```python
from build123d import *

# Parameters (mm, degrees)
SKETCH066_R     = 2.7
PAD030_DEPTH    = 10
SKETCH063_R     = 2.6
POCKET025_DEPTH = 8
SKETCH064_R     = 3
POCKET026_DEPTH = 1
SKETCH067_R     = 2
POCKET027_DEPTH = 8


with BuildPart() as loft003:
    # Sketch066 → Loft003 section 0
    with BuildSketch(Plane.XY.offset(18)):
        with Locations((-5, 0)):
            Circle(SKETCH066_R)
    # Sketch065 → Loft003 section 1
    with BuildSketch(Plane.XY.offset(38)):
        with BuildLine():
            ThreePointArc((-6, 1.5), (-7.5, 0), (-6, -1.5))
            Line((-6, -1.5), (-2, -1.5))
            ThreePointArc((-2, -1.5), (-0.5, 0), (-2, 1.5))
            Line((-2, 1.5), (-6, 1.5))
        make_face()
    loft()


with BuildPart() as part_mirroring003:
    # Part__Mirroring003: instance of Loft003
    add(loft003.part.mirror(Plane(origin=(0, 0, 0), x_dir=(0, -1, 0), z_dir=(1, 0, 0))))


with BuildPart() as fusion003:
    # Fusion003 base: copy of Loft003
    add(loft003.part)

    # Fusion003: union Part__Mirroring003
    add(part_mirroring003.part)


with BuildPart() as cut002:
    # Sketch062 → Pad030 (new body)
    with BuildSketch(Plane.XZ):
        Polygon((-16, 4), (-9.85, 4), (-9.85, 7), (-9.85, 8.6), (-9, 8.6), (-9, 10.6), (9, 10.6), (9, 8.6), (9.85, 8.6), (9.85, 7), (9.85, 4), (16, 4), (16, 12), (12.15, 15.85), (12.15, 26.306086), (16.15, 30), (16.15, 38), (-16.15, 38), (-16.15, 30), (-12.15, 26.306086), (-12.15, 15.85), (-16, 12), align=None)
    extrude(amount=PAD030_DEPTH)

    # Sketch063 (on Face7 of Pad030) → Pocket025 (cut)
    with BuildSketch(Plane(origin=(0, 0, 10.6), x_dir=(1, 0, 0), z_dir=(0, 0, -1))):
        with Locations((-5, 5)):
            Circle(SKETCH063_R)
        with Locations((5, 5)):
            Circle(SKETCH063_R)
    extrude(amount=-POCKET025_DEPTH, mode=Mode.SUBTRACT)

    # Sketch064 (on Face11 of Pocket025) → Pocket026 (cut)
    with BuildSketch(Plane(origin=(0, 0, 10.6), x_dir=(1, 0, 0), z_dir=(0, 0, -1))):
        with Locations((-5, 5)):
            Circle(SKETCH064_R)
        with Locations((5, 5)):
            Circle(SKETCH064_R)
    extrude(amount=-POCKET026_DEPTH, mode=Mode.SUBTRACT)

    # Sketch067 (on Face22 of Pocket026) → Pocket027 (cut)
    with BuildSketch(Plane(origin=(0, 0, 38), x_dir=(-1, 0, 0), z_dir=(0, 0, 1))):
        with Locations((-12, 5)):
            Circle(SKETCH067_R)
        with Locations((12, 5)):
            Circle(SKETCH067_R)
    extrude(amount=-POCKET027_DEPTH, mode=Mode.SUBTRACT)


with BuildPart() as cut002_1:
    # Body024 placement: moved
    add(cut002.part.moved(Location((0, 5, 0))))

    # Cut002: cut Fusion003
    add(fusion003.part, mode=Mode.SUBTRACT)


with BuildPart() as cut002_2:
    # Cut002 placement: moved
    add(cut002_1.part.moved(Location((0, -196.33, 0))))


solid = cut002_2.part
```
Work out the finished part from the listing and answer in its coordinate system (mm). A direction names the side the tool comes from. Round coordinates to 2 decimals unless told otherwise and drop trailing zeros. Loops run counter-clockwise (first coordinate to the right, second up) from the corner with the lowest first, then second, coordinate; pieces in that order, holes last.
(1) Each of these flat-tipped pins is pushed along its axis until it touches: P1, Ø2.5, axis at y = -197, z = 9, coming from the +X side; P2, Ø3, axis at x = 6, y = -195, coming from the -Z side; P3, Ø5, axis at y = -197.5, z = 20, coming from the +X side. Where does it stop, or does it pass through?
Computed values:
P1: stops at x = 16
P2: stops at z = 10.6
P3: stops at x = 12.15
(2) For faces 1 (the cylindrical face through (-2.6, -195.33, 14.76)), 2 (the cylindrical face through (11.077, -194.556, 34.056)), 3 (the flat face through (9.85, -196, 6)), determine the directions among +Z, -Z, +X, -X, +Y, -Y from which every point of the face is accessible in a straight line to the end or side of a thin tool.
Computed values:
face 1: -Z
face 2: +Z
face 3: -Z, +Y, -Y
(3) The part is cut by section A-A, the plane z = 15. Give the vertices of the cut face in (x, y), and give its area (3 significant figures).
Computed values:
outline: (-13, -201.33) - (13, -201.33) - (13, -191.33) - (-13, -191.33) - close; hole circle Ø5.2 at (-5, -196.33); hole circle Ø5.2 at (5, -196.33)
area: 218 mm2
(4) The part is cut by section B-B, the plane y = -192. Give the vertices of the cut face in (x, z).
Computed values:
outline: (-16.15, 30) - (-12.15, 26.31) - (-12.15, 15.85) - (-16, 12) - (-16, 4) - (-9.85, 4) - (-9.85, 8.6) - (-9, 8.6) - (-9, 10.6) - (9, 10.6) - (9, 8.6) - (9.85, 8.6) - (9.85, 4) - (16, 4) - (16, 12) - (12.15, 15.85) - (12.15, 26.31) - (16.15, 30) - (16.15, 38) - (-16.15, 38) - close
(5) The part is cut by section D-D, the plane z = 11. Give the vertices of the cut face in (x, y).
Computed values:
outline: (-16, -201.33) - (16, -201.33) - (16, -191.33) - (-16, -191.33) - close; hole circle Ø6 at (-5, -196.33); hole circle Ø6 at (5, -196.33)
(6) Find the intervals of material crossed by L1, parallel to X at y = -196.33, z = 10.9; L2, parallel to X at y = -192.25, z = 8; L3, parallel to Y at x = -5, z = 14, in increasing order.
Computed values:
L1: x = -16 to -8, -2 to 2, 8 to 16
L2: x = -16 to -9.85, 9.85 to 16
L3: y = -201.33 to -198.93, -193.73 to -191.33
(7) The mould has two halves that part along Z. Classify faces 4 (the flat face through (14.122, -196.26, 28.127)), 5 (the flat face through (12, -196, 30)), 6 (the cylindrical face through (4.609, -199.304, 11.093)): pulls with the +Z half, pulls with the -Z half, needs draft (parallel to the pull), parting line crosses it, or undercut.
Computed values:
face 4: undercut
face 5: pulls with the +Z half
face 6: needs draft
(8) The part is cut by section C-C, the plane x = 11. Give the vertices of the cut face in (y, z).
Computed values:
outline: (-201.33, 4) - (-191.33, 4) - (-191.33, 38) - (-194.6, 38) - (-194.6, 30) - (-198.06, 30) - (-198.06, 38) - (-201.33, 38) - close
